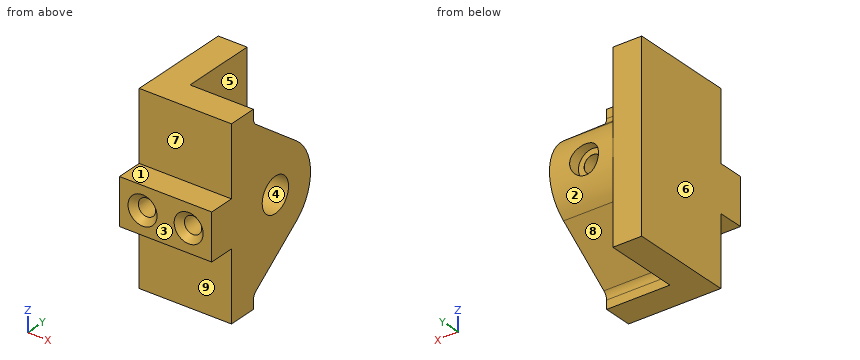
from build123d import *

# Parameters (mm, degrees)
BOSS_EXTRUDE1_DEPTH = 10
BOSS_EXTRUDE2_DEPTH = 22
SKETCH3_R           = 6
CUT_EXTRUDE1_DEPTH  = 24
LPATTERN1_COUNT     = 2
LPATTERN1_PITCH     = 16
FILLET1_R           = 3


# Read off the part's stored shape, not the designer's step: CBORE for M5 Hex Head Bolt1
with BuildPart() as part:
    # Sketch1 → Boss-Extrude1 (new body)
    with BuildSketch(Plane(origin=(0, 0, 0), x_dir=(0, 0, -1), z_dir=(1, 0, 0))):
        Polygon((-8, 0), (8, 0), (8, 9), (32, 9), (32, 45), (-32, 45), (-32, 9), (-8, 9), align=None)
    extrude(amount=BOSS_EXTRUDE1_DEPTH)

    # Sketch2 → Boss-Extrude2 (add)
    with BuildSketch(Plane(origin=(10, 0, 0), x_dir=(0, 0, -1), z_dir=(1, 0, 0))):
        with BuildLine():
            Line((-32, 9), (-32, 19))
            Line((-32, 19), (-27.5, 19))
            Line((-27.5, 19), (-12.799996672, 38.599999783))
            ThreePointArc((-12.799996672, 38.599999783), (0, 44.999997208), (12.799996672, 38.599999783))
            Line((12.799996672, 38.599999783), (27.5, 19))
            Line((27.5, 19), (32, 19))
            Line((32, 19), (32, 9))
            Line((32, 9), (8, 9))
            Line((8, 9), (8, 0))
            Line((8, 0), (-8, 0))
            Line((-8, 0), (-8, 9))
            Line((-8, 9), (-32, 9))
        make_face()
    extrude(amount=BOSS_EXTRUDE2_DEPTH)

    # Sketch3 → Cut-Extrude1 (cut)
    with BuildSketch(Plane(origin=(32, 0, 0), x_dir=(0, 0, -1), z_dir=(1, 0, 0))):
        with Locations((0, 29)):
            Circle(SKETCH3_R)
    extrude(amount=-CUT_EXTRUDE1_DEPTH, mode=Mode.SUBTRACT)

    # CBORE for M5 Hex Head Bolt1 outline → CBORE for M5 Hex Head Bolt1 (revolve, cut)
    with BuildSketch(Plane(origin=(20, 0, 0), x_dir=(1, 0, 0), z_dir=(0, 0, 1))):
        Polygon((3.025, 41), (5, 41), (5, 44.975), (5.025014792, 45.000014792), (0, 45.000014792), (0, 34.195854076), (3, 34.195854076), (3, 40.975), align=None)
    revolve(axis=Axis((20, 0, 0), (0, 1, 0)), mode=Mode.SUBTRACT)

    # Sketch9 → Ø1.0mm Dowel Hole1 (revolve, cut)
    with BuildSketch(Plane(origin=(24, 0, 0), x_dir=(0, 0, -1), z_dir=(1, 0, 0))):
        Polygon((0, 0), (0, 17.732050808), (3, 16), (3, 2.025), (5.025, 0), align=None)
    f_1_0mm_dowel_hole1 = revolve(axis=Axis((24, -6.35, 0), (0, 1, 0)), mode=Mode.SUBTRACT)

    # LPattern1: Ø1.0mm Dowel Hole1 ×2
    with Locations(*[(-i * LPATTERN1_PITCH, 0, 0) for i in range(1, LPATTERN1_COUNT)]):
        add(f_1_0mm_dowel_hole1, mode=Mode.SUBTRACT)

    # Fillet1
    fillet1_edges = [part.edges().sort_by_distance(p)[0] for p in [
        (21, 19, 27.5),
        (21, 19, -27.5),
    ]]
    fillet(fillet1_edges, radius=FILLET1_R)


solid = part.part
Geometry: final body of the model. Coordinates: model frame, mm. Face numbers are marked on the shaded views. A direction names the side the tool comes from. Round coordinates to 2 decimals unless told otherwise and drop trailing zeros. Order: outer loops, then holes, each group sorted by start corner. A loop starts at its lowest first (then second) coordinate and runs counter-clockwise, first axis right, second up. Notation, with made-up numbers: (-29, 2.5) -> (-22, 2.5) arc R19 cw to (-22, 8.5) -> close; hole circle Ø8 at (89.25, -34). An arc over 180 degrees is marked (long way). Put each result on its own line as item: value. Start each with the question number.
Q1. Reachability of the marked faces 5, 6, 7, 8 and 9 from +Z, -Z, +X, -X, +Y, -Y: full face, straight path, thin tool, end or side. Return the list, or none.
Q2. First-contact query: pin 1 (5 mm diameter, centred on x = 20, z = 0, fed in from +Y); pin 2 (3.5 mm diameter, centred on x = 24, z = 0, fed in from -Y); pin 3 (7 mm diameter, centred on x = 14.5, y = 4, fed in from -Z). Flat tips, straight axial feed; report the tip coordinate or a pass-through.
Q3. Section C-C on z = -16.5. Return the cut outline in (x, y).
Q4. Section D-D on x = 16. Return the cut outline in (y, z), and give its area (3 significant figures).
Q5. Section A-A on x = 30.5. Return the cut outline in (y, z), and give its area (3 significant figures).
Q6. Pull-direction query (Z, two-part tool) for the marked faces 1, 2, 3 and 4; classes: +Z half, -Z half, draft (parallel to the pull), parting line (faces both ways), or undercut.
Q7. Section B-B on y = 10.5. Return the cut outline in (x, z).
Q8. Line query: probe 1 along X at (y, z) = (11, 0); probe 2 along Z at (x, y) = (8, 11); probe 3 along Z at (x, y) = (8, 7.5). Output: solid intervals per line, ascending.
Ans:
1. face 5: +X, +Y
1. face 6: +Z, -Z, -X, +Y, -Y
1. face 7: +Z, +X, -X, -Y
1. face 8: -Z, +X, +Y
1. face 9: -Z, +X, -X, -Y
2. pin 1: stops at y = 23.55
2. pin 2: stops at y = 16.72
2. pin 3: stops at z = -8
3. outline: (0, 9) -> (32, 9) -> (32, 33.67) -> (10, 33.67) -> (10, 45) -> (0, 45) -> close
4. outline: (0, -8) -> (9, -8) -> (9, -32) -> (19, -32) -> (19, -29) arc R3 cw to (20.2, -26.6) -> (38.6, -12.8) arc R16 ccw to (44.72, -3) -> (41, -3) -> (41, 3) -> (44.72, 3) arc R16 ccw to (38.6, 12.8) -> (20.2, 26.6) arc R3 cw to (19, 29) -> (19, 32) -> (9, 32) -> (9, 8) -> (0, 8) -> close; hole circle Ø12 at (29, 0)
4. area: 1,550 mm2
5. outline: (0, -8) -> (9, -8) -> (9, -32) -> (19, -32) -> (19, -29) arc R3 cw to (20.2, -26.6) -> (38.6, -12.8) arc R16 ccw to (38.6, 12.8) -> (20.2, 26.6) arc R3 cw to (19, 29) -> (19, 32) -> (9, 32) -> (9, 8) -> (0, 8) -> close; hole circle Ø12 at (29, 0)
5. area: 1,580 mm2
6. face 1: +Z half
6. face 2: parting line
6. face 3: draft
6. face 4: undercut
7. outline: (0, -32) -> (32, -32) -> (32, 32) -> (0, 32) -> close; hole circle Ø6 at (8, 0); hole circle Ø6 at (24, 0)
8. probe 1: x = 0 to 5, 11 to 21, 27 to 32
8. probe 2: z = -32 to -3, 3 to 32
8. probe 3: z = -8 to -3, 3 to 8
